Job drawing, mm, ordinate dimensions from the low corner. One solid piece. A direction names the side the tool comes from. Coordinates: 2 decimals unless noted, no trailing zeros. Write each loop counter-clockwise with the first axis right and the second up, starting at its lowest first coordinate (ties: lowest second). Pieces come first, ordered by that corner, then holes. Notation, with made-up numbers: (13, -26) - (64, -26) arc R13 ccw to (64, -9) - close; hole circle Ø6 at (-13.75, -20). An arc over 180 degrees is marked (long way). Use a Markdown table: item, result.
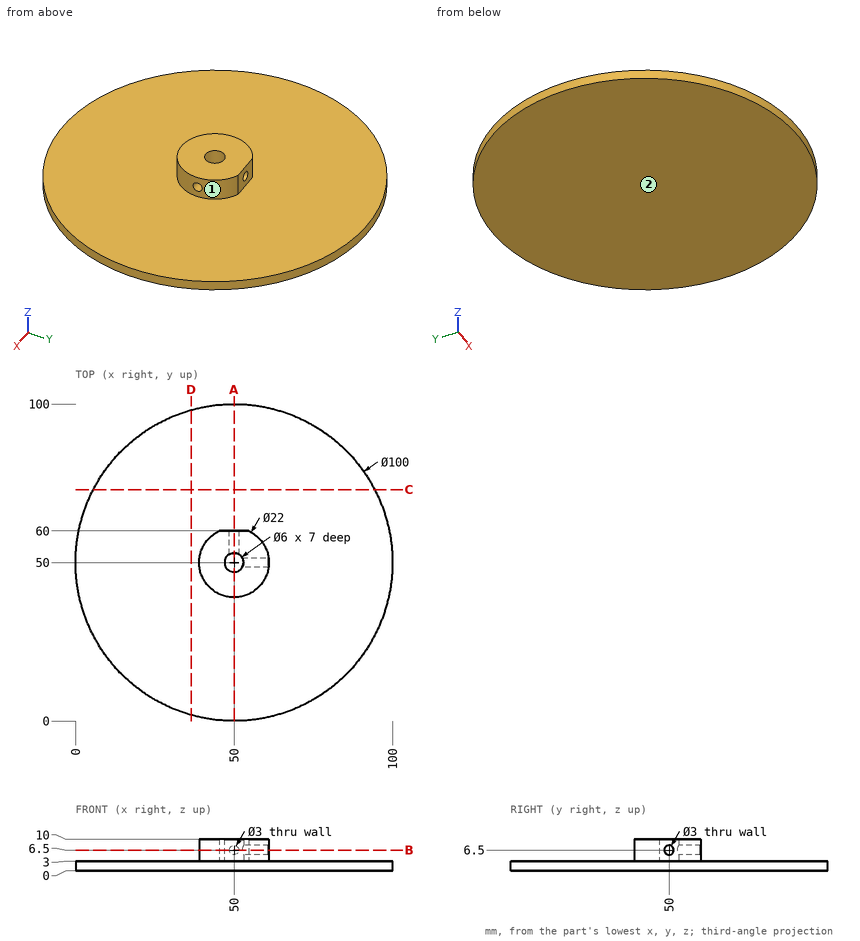
Item 1: Band-saw the part on D-D, the plane x = 36.5. Give the cut face in (y, z), then the cut area to 3 significant figures.
From the geometry:
| item | result |
|---|---|
| outline | (1.86, 0) - (98.14, 0) - (98.14, 3) - (1.86, 3) - close |
| area | 289 mm^2 |
Item 2: Band-saw the part on B-B, the plane z = 6.5. Give the cut face in (x, y), then the cut area to 3 significant figures.
From the geometry:
| item | result |
|---|---|
| outline | (45.42, 60) arc R11 ccw (long way) to (60.9, 48.5) - (52.6, 48.5) arc R3 cw (long way) to (48.5, 52.6) - (48.5, 60) - close; (51.5, 52.6) arc R3 cw to (52.6, 51.5) - (60.9, 51.5) arc R11 ccw to (54.58, 60) - (51.5, 60) - close |
| area | 300 mm^2 |
Item 3: Drill centre lines: probe 1 along Z at (x, y) = (57.75, 50); probe 2 along Z at (x, y) = (80.5, 55); probe 3 along X at (y, z) = (55.5, 6.5). Where is each one in solid material? Low to high.
From the geometry:
| item | result |
|---|---|
| probe 1 | 0 to 5, 8 to 10 |
| probe 2 | 0 to 3 |
| probe 3 | 40.47 to 48.5, 51.5 to 59.53 |
Item 4: Drop flat-ended pins along their axis: P1, Ø8, axis at x = 27, y = 81.5, coming from the +Z side; P2, Ø1.8, axis at x = 50, z = 6.5, coming from the +Y side; P3, Ø6, axis at x = 87, z = 1.5, coming from the -Y side. Give the stop position or say it passes through.
From the geometry:
| item | result |
|---|---|
| P1 | z = 3 |
| P2 | y = 47.14 |
| P3 | y = 13.34 |
Item 5: Which spindle directions (+Z, -Z, +X, -X, +Y, -Y) get a long thin tool onto all of the face, cutting with end or side? Do the marked faces 1 and 2. Say none if no direction does.
From the geometry:
| item | result |
|---|---|
| face 1 | +Z |
| face 2 | -Z, +X, -X, +Y, -Y |
Item 6: Band-saw the part on C-C, the plane y = 73. Give the cut face in (x, z), then the cut area to 3 significant figures.
From the geometry:
| item | result |
|---|---|
| outline | (5.6, 0) - (94.4, 0) - (94.4, 3) - (5.6, 3) - close |
| area | 266 mm^2 |
Item 7: Band-saw the part on A-A, the plane x = 50. Give the cut face in (y, z).
From the geometry:
| item | result |
|---|---|
| outline | (0, 0) - (100, 0) - (100, 3) - (60, 3) - (60, 5) - (53, 5) - (53, 3) - (47, 3) - (47, 10) - (39, 10) - (39, 3) - (0, 3) - close; (53, 8) - (60, 8) - (60, 10) - (53, 10) - close |
